```python
from build123d import *

# Parameters (mm, degrees)
F1_DEPTH = 6.35
F2_R     = 12.7
F2_R_2   = 9.525
F2_R_3   = 2.38125
F3_DEPTH = 1.5875
F4_W     = 3.175
F4_H     = 25.4
F5_DEPTH = 3.175
F6_W     = 38.1
F6_H     = 25.4
F7_DEPTH = 3.175


with BuildPart() as f1:
    # F0 (on Top) → F1 (new body)
    with BuildSketch(Plane.XY):
        Polygon((-6.35, 0), (-50.8, 0), (-57.15, -6.35), (-57.15, -50.8), (-50.8, -57.15), (-6.35, -57.15), (0, -50.8), (0, -6.35), align=None)
    extrude(amount=F1_DEPTH)

    # F2 (on face) → F3 (join)
    with BuildSketch(Plane.XY.offset(6.35)):
        Polygon((0, -6.35), (-6.35, 0), (-50.8, 0), (-57.15, -6.35), (-57.15, -50.8), (-50.8, -57.15), (-6.35, -57.15), (0, -50.8), align=None)
        Polygon((-3.175, -7.665128), (-3.175, -49.484872), (-7.665128, -53.975), (-49.484872, -53.975), (-53.975, -49.484872), (-53.975, -7.665128), (-49.484872, -3.175), (-7.665128, -3.175), align=None, mode=Mode.SUBTRACT)
        with BuildLine():
            Line((-28.575, -52.3875), (-24.084872, -47.897372))
            ThreePointArc((-24.084872, -47.897372), (-9.252628, -47.897372), (-9.252628, -33.065128))
            Line((-9.252628, -33.065128), (-4.7625, -28.575))
            Line((-4.7625, -28.575), (-9.252628, -24.084872))
            ThreePointArc((-9.252628, -24.084872), (-9.252628, -9.252628), (-24.084872, -9.252628))
            Line((-24.084872, -9.252628), (-28.575, -4.7625))
            Line((-28.575, -4.7625), (-33.065128, -9.252628))
            ThreePointArc((-33.065128, -9.252628), (-47.897372, -9.252628), (-47.897372, -24.084872))
            Line((-47.897372, -24.084872), (-52.3875, -28.575))
            Line((-52.3875, -28.575), (-47.897372, -33.065128))
            ThreePointArc((-47.897372, -33.065128), (-47.897372, -47.897372), (-33.065128, -47.897372))
            Line((-33.065128, -47.897372), (-28.575, -52.3875))
        make_face()
        with BuildLine():
            ThreePointArc((-23.572089, -14.255539), (-11.497692, -11.497692), (-14.255539, -23.572089))
            Line((-14.255539, -23.572089), (-9.252628, -28.575))
            Line((-9.252628, -28.575), (-14.255539, -33.577911))
            ThreePointArc((-14.255539, -33.577911), (-11.497692, -45.652308), (-23.572089, -42.894461))
            Line((-23.572089, -42.894461), (-28.575, -47.897372))
            Line((-28.575, -47.897372), (-33.577911, -42.894461))
            ThreePointArc((-33.577911, -42.894461), (-45.652308, -45.652308), (-42.894461, -33.577911))
            Line((-42.894461, -33.577911), (-47.897372, -28.575))
            Line((-47.897372, -28.575), (-42.894461, -23.572089))
            ThreePointArc((-42.894461, -23.572089), (-45.652308, -11.497692), (-33.577911, -14.255539))
            Line((-33.577911, -14.255539), (-28.575, -9.252628))
            Line((-28.575, -9.252628), (-23.572089, -14.255539))
        make_face(mode=Mode.SUBTRACT)
        with Locations((-28.575, -28.575)):
            Circle(F2_R)
        with Locations((-28.575, -28.575)):
            Circle(F2_R_2, mode=Mode.SUBTRACT)
        with Locations((-40.48125, -40.48125)):
            Circle(F2_R_3)
        with Locations((-16.66875, -40.48125)):
            Circle(F2_R_3)
        with Locations((-16.66875, -16.66875)):
            Circle(F2_R_3)
        with Locations((-40.48125, -16.66875)):
            Circle(F2_R_3)
    extrude(amount=F3_DEPTH)

    # F4 (on face) → F5 (join)
    with BuildSketch(Plane(origin=(0, 0, 0), x_dir=(1, 0, 0), z_dir=(0, 0, -1))):
        with Locations((-46.0375, 28.575)):
            Rectangle(F4_W, F4_H)
        with Locations((-11.1125, 28.575)):
            Rectangle(F4_W, F4_H)
    extrude(amount=F5_DEPTH)

    # F6 (on face) → F7 (join)
    with BuildSketch(Plane(origin=(0, 0, -3.175), x_dir=(1, 0, 0), z_dir=(0, 0, -1))):
        with Locations((-28.575, 28.575)):
            Rectangle(F6_W, F6_H)
    extrude(amount=F7_DEPTH)


solid = f1.part
```
Geometry check sheet. Reference: the model listing, model coordinates, mm. A direction names the side the tool comes from. Give positions to 0.01 mm unless a question says otherwise; leave off trailing zeros. Loops run counter-clockwise (first coordinate to the right, second up) from the corner with the lowest first, then second, coordinate; pieces in that order, holes last. Notation, with made-up numbers: (38, -36) - (44, -36) arc R17 cw to (44, -31) - close; hole circle Ø5 at (48, 82). An arc over 180 degrees is marked (long way). Use CSV: the item, a comma, the result in double quotes. Start each with the question number.
Q1. Go/stop test with flat-tipped pins: pin 1 Ø1.6 at (y, z) = (-29.5, -2.5) entering from -X (3 decimals); pin 2 Ø5 at (x, z) = (-16.5, -2) entering from -Y; pin 3 Ø9.5 at (x, y) = (-32, -31.5) entering from +Z; pin 4 Ø1.9 at (x, z) = (-22, -4) entering from -Y (3 decimals). Record where each tip stops, or that it passes through.
Q2. Release check for a two-part mould opening along X. For faces 4 (the face through (-29, -41.275, -5)), 5 (the face through (-57.15, -28, 4)), 6 (the face through (-7.04, -30.85, 7.13)) record: +X half, -X half, draft (parallel to the pull), parting line (faces both ways), or undercut.
Q3. Access from +Z, -Z, +X, -X, +Y, -Y to the whole of each face (thin tool, end or side, straight path). Record for faces 1 (the face through (-29, -3.175, 7)), 2 (the face through (-12.7, -28, -2)), 3 (the face through (-29, -29, -6.35)).
Q4. Scan lines: probe 1 along Z at (x, y) = (-16, -19) (3 decimals); probe 2 along Y at (x, z) = (-10.5, 6.75) (3 decimals); probe 3 along Z at (x, y) = (-13, -4). Record each from-to range of solid material in increasing order. Write a range as from..to.
Q5. Section check A-A, the plane z = -1.75. Record the cut outline in (x, y) (3 decimals).
Findings below:
1,pin 1,"stops at x = -47.625"
1,pin 2,"stops at y = -57.15"
1,pin 3,"stops at z = 6.35"
1,pin 4,"stops at y = -41.275"
2,face 4,"draft"
2,face 5,"-X half"
2,face 6,"undercut"
3,face 1,"+Z"
3,face 2,"+Y, -Y"
3,face 3,"-Z, +X, -X, +Y, -Y"
4,probe 1,"z = -6.35..-3.175, 0..6.35"
4,probe 2,"y = -57.15..-53.975, -48.963..-44.409, -36.554..-29.822, -27.328..-20.596, -12.741..-8.187, -3.175..0"
4,probe 3,"z = 0..6.35"
5,outline,"(-47.625, -41.275) - (-44.45, -41.275) - (-44.45, -15.875) - (-47.625, -15.875) - close; (-12.7, -41.275) - (-9.525, -41.275) - (-9.525, -15.875) - (-12.7, -15.875) - close"
